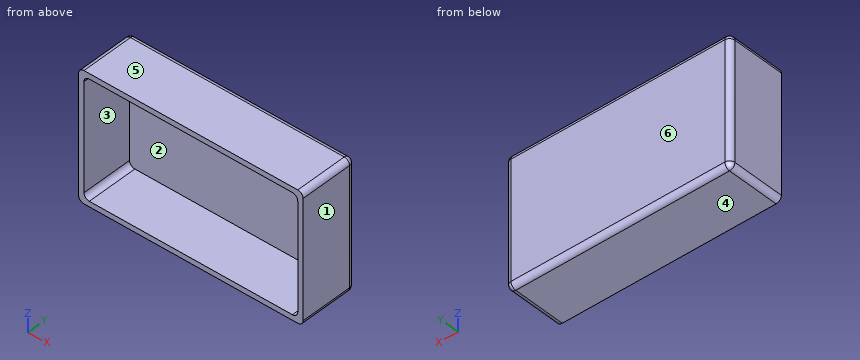
```python
from build123d import *

# Parameters (mm, degrees)
F0_W        = 105
F0_H        = 60
F0_W_2      = 100
F0_H_2      = 55
F2_DEPTH    = 24
F2_FACE_W   = 105
F2_FACE_H   = 60
F2_FACE_W_2 = 100
F2_FACE_H_2 = 55
F1_R        = 3
F1_R_2      = 1.25
F3_DEPTH    = 3
F4_R        = 2.5


with BuildPart() as f2:
    # F0 (on Front) → F2 (new body)
    with BuildSketch(Plane.XZ):
        Rectangle(F0_W, F0_H)
        Rectangle(F0_W_2, F0_H_2, mode=Mode.SUBTRACT)
    extrude(amount=F2_DEPTH)

    # F0 (on Front) + F2_face (on face) + F1 (on Front) → F3 (join)
    with BuildSketch(Plane.XZ):
        Rectangle(F0_W_2, F0_H_2)
    with BuildSketch(Plane.XZ.offset(24)):
        Rectangle(F2_FACE_W, F2_FACE_H)
        Rectangle(F2_FACE_W_2, F2_FACE_H_2, mode=Mode.SUBTRACT)
    with BuildSketch(Plane.XZ):
        with Locations((-42.9925474213, -21.9911143348)):
            Circle(F1_R)
        with Locations((-42.9925474213, -21.9911143348)):
            Circle(F1_R_2, mode=Mode.SUBTRACT)
        with Locations((-42.9925474213, 22.0088856652)):
            Circle(F1_R)
        with Locations((-42.9925474213, 22.0088856652)):
            Circle(F1_R_2, mode=Mode.SUBTRACT)
        with Locations((43.0074525787, 22.0088856652)):
            Circle(F1_R)
        with Locations((43.0074525787, 22.0088856652)):
            Circle(F1_R_2, mode=Mode.SUBTRACT)
        with Locations((43.0074525787, -21.9911143348)):
            Circle(F1_R)
        with Locations((43.0074525787, -21.9911143348)):
            Circle(F1_R_2, mode=Mode.SUBTRACT)
    extrude(amount=F3_DEPTH)

    # F4
    f4_edges = [f2.edges().sort_by_distance(p)[0] for p in [
        (-52.5, -13.5, -30),
        (52.5, -13.5, -30),
        (52.5, -13.5, 30),
        (-52.5, -13.5, 30),
        (0, 0, 30),
        (-52.5, 0, 0),
        (0, 0, -30),
        (52.5, 0, 0),
        (50, -15, -27.5),
        (-50, -15, -27.5),
        (50, -15, 27.5),
        (-50, -15, 27.5),
    ]]
    fillet(f4_edges, radius=F4_R)


solid = f2.part
```
CAD build for the part. Positions are in the model's coordinates, mm. Face numbers are marked on the shaded views. A direction names the side the tool comes from. Round coordinates to 2 decimals unless told otherwise and drop trailing zeros. Write each loop counter-clockwise with the first axis right and the second up, starting at its lowest first coordinate (ties: lowest second). Pieces come first, ordered by that corner, then holes.
Item 1: Band-saw the part on A-A on y = -6.25. Write the cut outline in (x, z).
Filled in:
outline: (-52.5, -27.5) arc R2.5 ccw to (-50, -30) - (50, -30) arc R2.5 ccw to (52.5, -27.5) - (52.5, 27.5) arc R2.5 ccw to (50, 30) - (-50, 30) arc R2.5 ccw to (-52.5, 27.5) - close; hole (-50, -25) arc R2.5 ccw to (-47.5, -27.5) - (47.5, -27.5) arc R2.5 ccw to (50, -25) - (50, 25) arc R2.5 ccw to (47.5, 27.5) - (-47.5, 27.5) arc R2.5 ccw to (-50, 25) - close
Item 2: Band-saw the part on C-C on x = 7.5. Write the cut outline in (y, z).
Filled in:
outline: (-27, -30) - (-2.5, -30) arc R2.5 ccw to (0, -27.5) - (0, 27.5) arc R2.5 ccw to (-2.5, 30) - (-27, 30) - (-27, 27.5) - (-3, 27.5) - (-3, -27.5) - (-27, -27.5) - close
Item 3: Drop a flat-ended pin along its axis: pin 1 Ø6 at (x, z) = (-26, -15.5) entering from -Y. Give the stop position or say it passes through.
Filled in:
pin 1: stops at y = -3
Item 4: Drill centre lines: L1, parallel to Z at x = -2.5, y = -13.25; L2, parallel to X at y = -22, z = -10; L3, parallel to Y at x = 8, z = 15. Where is each one in solid material? Low to high.
Filled in:
L1: z = -30 to -27.5, 27.5 to 30
L2: x = -52.5 to -50, 50 to 52.5
L3: y = -3 to 0
Item 5: Mould opens along Z. For the marked faces 3, 4, 5 and 6 say: released by +Z, released by -Z, zero draft, split by the parting line, or undercut.
Filled in:
face 3: undercut
face 4: released by -Z
face 5: released by +Z
face 6: zero draft
Item 6: Tool access for the marked faces 1 and 2: list every direction of +Z, -Z, +X, -X, +Y, -Y with a clear straight run to the whole face (end or side of a thin tool).
Filled in:
face 1: +Z, -Z, +X, +Y, -Y
face 2: -Y
Item 7: Band-saw the part on B-B on z = 6.5. Write the cut outline in (x, y), then the cut area to 3 significant figures.
Filled in:
outline: (-52.5, -27) - (-50, -27) - (-50, -3) - (50, -3) - (50, -27) - (52.5, -27) - (52.5, -2.5) arc R2.5 ccw to (50, 0) - (-50, 0) arc R2.5 ccw to (-52.5, -2.5) - close
area: 432 mm2
